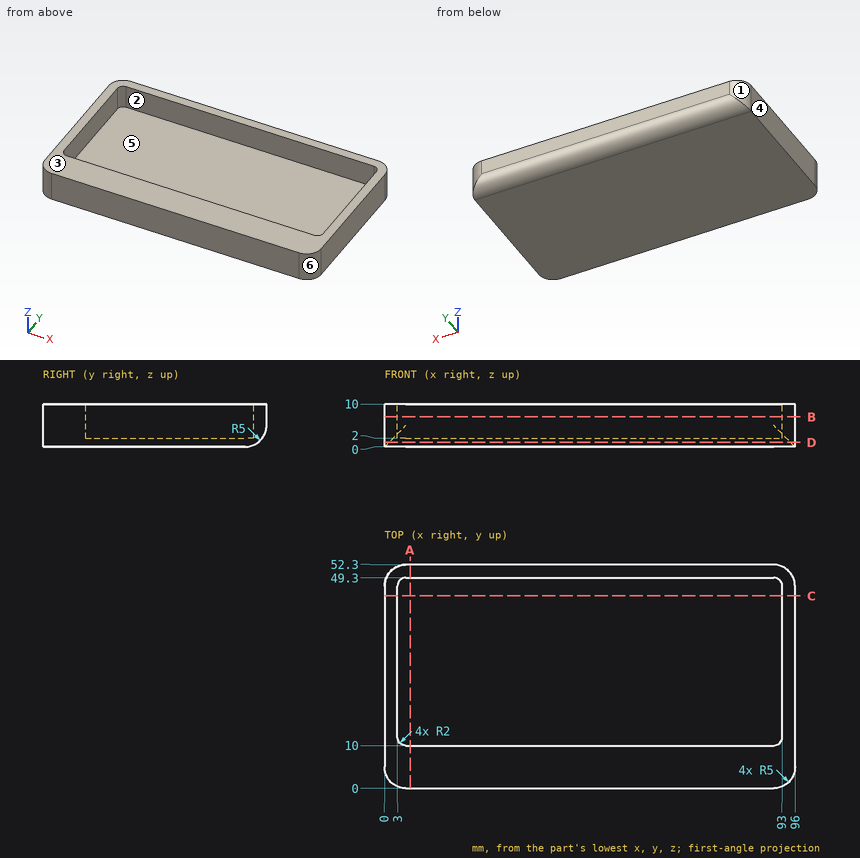
Could you check a few things on this drawing? It's one solid part, dimensions in mm from its lowest x, y, z. A direction names the side the tool comes from. Give positions to 0.01 mm unless a question says otherwise; leave off trailing zeros. Write each loop counter-clockwise with the first axis right and the second up, starting at its lowest first coordinate (ties: lowest second). Pieces come first, ordered by that corner, then holes. Notation, with made-up numbers: (72.25, 29) -> (87.25, 29) arc R19 ccw to (87.25, 35) -> close; hole circle Ø10 at (-11.75, 11.25). An arc over 180 degrees is marked (long way). Answer as CSV lines item,"result". Start each with the question number.
(1) If we mould it in two halves opening along X, with no side actions, what happens to the marked faces 3, 4, 5 and 6? For each: +X half, -X half, draft (parallel to the pull), parting line (faces both ways), or undercut.
(2) If we section it at D-D, the plane z = 1: Write out the boundary of the cut face in (x, y), and give its area (3 significant figures).
(3) If we section it at C-C, the plane y = 45: Write out the boundary of the cut face in (x, z), and give its area (3 significant figures).
(4) If we section it at B-B, the plane z = 7: Write out the boundary of the cut face in (x, y), and give its area (3 significant figures).
(5) Which directions (+Z, -Z, +X, -X, +Y, -Y) give clear straight access to the entire face, cutting with the end or side of a thin tool? Please do the marked faces 1 and 2.
(6) Please list where these lines run through material, in increasing order: line 1 (Y direction, x = 11.5, z = 5.5); line 2 (X direction, y = 38, z = 2.25); line 3 (Z direction, x = 91.5, y = 32.5).
(7) I'm going to push a flat-ended pin straight in: pin 1 Ø2 at (x, y) = (24, 36) entering from +Z. Where does the tip first touch, or does it pass through?
(8) If we section it at A-A, the plane x = 6: Write out the boundary of the cut face in (y, z).
Answer list:
1,face 3,"draft"
1,face 4,"-X half"
1,face 5,"undercut"
1,face 6,"+X half"
2,outline,"(0, 5) arc R5 ccw to (5, 0) -> (91, 0) arc R5 ccw to (96, 5) -> (96, 47.3) arc R5 ccw to (95, 50.3) -> (1, 50.3) arc R5 ccw to (0, 47.3) -> close"
2,area,"4,820 mm^2"
3,outline,"(0, 0) -> (96, 0) -> (96, 10) -> (93, 10) -> (93, 2) -> (3, 2) -> (3, 10) -> (0, 10) -> close"
3,area,"240 mm^2"
4,outline,"(0, 5) arc R5 ccw to (5, 0) -> (91, 0) arc R5 ccw to (96, 5) -> (96, 47.3) arc R5 ccw to (91, 52.3) -> (5, 52.3) arc R5 ccw to (0, 47.3) -> close; hole (3, 12) arc R2 ccw to (5, 10) -> (91, 10) arc R2 ccw to (93, 12) -> (93, 47.3) arc R2 ccw to (91, 49.3) -> (5, 49.3) arc R2 ccw to (3, 47.3) -> close"
4,area,"1,470 mm^2"
5,face 1,"+Z, -Z, -X, +Y"
5,face 2,"+Z"
6,line 1,"0 to 10, 49.3 to 52.3"
6,line 2,"0 to 3, 93 to 96"
6,line 3,"0 to 2"
7,pin 1,"z = 2"
8,outline,"(0, 0) -> (47.3, 0) arc R5 ccw to (52.3, 5) -> (52.3, 10) -> (49.3, 10) -> (49.3, 2) -> (10, 2) -> (10, 10) -> (0, 10) -> close"
